Model file for the job. Use its own axes, mm. A direction names the side the tool comes from. Round coordinates to 2 decimals unless told otherwise and drop trailing zeros. Loops run counter-clockwise (first coordinate to the right, second up) from the corner with the lowest first, then second, coordinate; pieces in that order, holes last. Notation, with made-up numbers: M 60.5,-22.5 L 67.5,-22.5 A23 ccw 67.5,6.5 Z; hole C -25,-2 d3. An arc over 180 degrees is marked long. Answer in a Markdown table with one row per item.
from build123d import *

# Parameters (mm, degrees)
SKETCH1_W           = 109.1
SKETCH1_H           = 40
BOSS_EXTRUDE1_DEPTH = 8
SKETCH2_W           = 22.3
SKETCH2_H           = 48
BOSS_EXTRUDE2_DEPTH = 8
SKETCH3_W           = 24.8
SKETCH3_H           = 40
BOSS_EXTRUDE3_DEPTH = 6
SKETCH4_R           = 2
CUT_EXTRUDE1_DEPTH  = 6.7
SKETCH5_R           = 2
CUT_EXTRUDE2_DEPTH  = 6.7
SKETCH6_R           = 2
CUT_EXTRUDE3_DEPTH  = 6.7


with BuildPart() as part:
    # Sketch1 → Boss-Extrude1 (new body)
    with BuildSketch(Plane.XY.offset(246)):
        with Locations((281.75, 300)):
            Rectangle(SKETCH1_W, SKETCH1_H)
        with BuildLine():
            Line((282, 296), (282, 304))
            ThreePointArc((282, 304), (280, 306), (278, 304))
            Line((278, 304), (278, 296))
            ThreePointArc((278, 296), (280, 294), (282, 296))
        make_face(mode=Mode.SUBTRACT)
        with BuildLine():
            Line((302, 296), (302, 304))
            ThreePointArc((302, 304), (300, 306), (298, 304))
            Line((298, 304), (298, 296))
            ThreePointArc((298, 296), (300, 294), (302, 296))
        make_face(mode=Mode.SUBTRACT)
    extrude(amount=BOSS_EXTRUDE1_DEPTH)

    # Sketch2 → Boss-Extrude2 (add)
    with BuildSketch(Plane.XY.offset(246)):
        with Locations((325.15, 300)):
            Rectangle(SKETCH2_W, SKETCH2_H)
    extrude(amount=BOSS_EXTRUDE2_DEPTH)

    # Sketch3 → Boss-Extrude3 (add)
    with BuildSketch(Plane.XY.offset(254)):
        with Locations((239.6, 300)):
            Rectangle(SKETCH3_W, SKETCH3_H)
    extrude(amount=BOSS_EXTRUDE3_DEPTH)

    # Sketch4 → Cut-Extrude1 (cut)
    with BuildSketch(Plane.XY.offset(253.3)):
        with Locations(Location((233, 288, 0), (0, 0, 180))):
            Circle(SKETCH4_R)
        with Locations(Location((233, 312, 0), (0, 0, 180))):
            Circle(SKETCH4_R)
        with Locations(Location((245, 288, 0), (0, 0, 180))):
            Circle(SKETCH4_R)
        with Locations(Location((245, 312, 0), (0, 0, 180))):
            Circle(SKETCH4_R)
    extrude(amount=CUT_EXTRUDE1_DEPTH, mode=Mode.SUBTRACT)

    # Sketch5 → Cut-Extrude2 (cut)
    with BuildSketch(Plane.XY.offset(247.3)):
        with Locations(Location((320, 282.7, 0), (0, 0, 180))):
            Circle(SKETCH5_R)
        with Locations(Location((320, 317.3, 0), (0, 0, 180))):
            Circle(SKETCH5_R)
        with Locations(Location((329.5, 282.7, 0), (0, 0, 180))):
            Circle(SKETCH5_R)
        with Locations(Location((329.5, 317.3, 0), (0, 0, 180))):
            Circle(SKETCH5_R)
    extrude(amount=CUT_EXTRUDE2_DEPTH, mode=Mode.SUBTRACT)

    # Sketch6 → Cut-Extrude3 (cut)
    with BuildSketch(Plane.XY.offset(246)):
        with Locations(Location((238, 294, 0), (0, 0, 180))):
            Circle(SKETCH6_R)
        with Locations(Location((238, 306, 0), (0, 0, 180))):
            Circle(SKETCH6_R)
        with Locations(Location((326, 292, 0), (0, 0, 180))):
            Circle(SKETCH6_R)
        with Locations(Location((326, 308, 0), (0, 0, 180))):
            Circle(SKETCH6_R)
    extrude(amount=CUT_EXTRUDE3_DEPTH, mode=Mode.SUBTRACT)


solid = part.part
1. Pin check, flat tips, straight feed: pin 1 (8 mm diameter, centred on x = 240.5, z = 252, fed in from -Y); pin 2 (2 mm diameter, centred on y = 277, z = 250.5, fed in from -X); pin 3 (5 mm diameter, centred on y = 299, z = 258.5, fed in from +X). Stop position of each tip, or through.
Verdict:
| item | result |
|---|---|
| pin 1 | stops at y = 280 |
| pin 2 | stops at x = 314 |
| pin 3 | stops at x = 252 |
2. Saw through at A-A (x = 300). Write the cut outline in (y, z), and give its area (3 significant figures).
Verdict:
| item | result |
|---|---|
| outline | M 280,246 L 294,246 L 294,254 L 280,254 Z; M 306,246 L 320,246 L 320,254 L 306,254 Z |
| area | 224 mm² |
3. Wall check: probe 1 along Y at (x, z) = (320, 250); probe 2 along Y at (x, z) = (233, 256.5); probe 3 along X at (y, z) = (288, 255). Give the ranges that are in metal, low to high.
Verdict:
| item | result |
|---|---|
| probe 1 | y = 276 to 280.7, 284.7 to 315.3, 319.3 to 324 |
| probe 2 | y = 280 to 286, 290 to 310, 314 to 320 |
| probe 3 | x = 227.2 to 231, 235 to 243, 247 to 252 |
4. Saw through at C-C (y = 305). Write the cut outline in (x, z), and give its area (3 significant figures).
Verdict:
| item | result |
|---|---|
| outline | M 227.2,246 L 236.27,246 L 236.27,252.7 L 239.73,252.7 L 239.73,246 L 278.27,246 L 278.27,254 L 252,254 L 252,260 L 227.2,260 Z; M 281.73,246 L 298.27,246 L 298.27,254 L 281.73,254 Z; M 301.73,246 L 336.3,246 L 336.3,254 L 301.73,254 Z |
| area | 943 mm² |
5. Saw through at D-D (z = 256.25). Write the cut outline in (x, y), and give its area (3 significant figures).
Verdict:
| item | result |
|---|---|
| outline | M 227.2,280 L 252,280 L 252,320 L 227.2,320 Z; hole C 233,288 d4; hole C 233,312 d4; hole C 245,288 d4; hole C 245,312 d4 |
| area | 942 mm² |
6. Mould opens along X. For faces 4 (the flat face through (325, 324, 250)), 5 (the flat face through (326, 308, 252.7)), 6 (the flat face through (314, 322, 250)) say: +X half, -X half, draft (parallel to the pull), parting line (faces both ways), or undercut.
Verdict:
| item | result |
|---|---|
| face 4 | draft |
| face 5 | undercut |
| face 6 | -X half |
7. Saw through at B-B (z = 250). State how many separate pieces and enclosed holes the cut face has, and give its area (3 significant figures).
Verdict:
| item | result |
|---|---|
| separate pieces | 1 |
| enclosed holes | 10 |
| area | 4,350 mm² |
8. Tool access for faces 1 (the cylindrical face through (331.1, 318.5, 250.6)), 2 (the flat face through (260, 280, 251)), 3 (the cylindrical face through (327.6, 293.2, 249.3)): list every direction of +Z, -Z, +X, -X, +Y, -Y with a clear straight run to the whole face (end or side of a thin tool).
Verdict:
| item | result |
|---|---|
| face 1 | +Z |
| face 2 | +Z, -Z, -X, -Y |
| face 3 | -Z |
